Input: part model. Units: mm. Frame: model coordinates. Face numbers are marked on the shaded views. A direction names the side the tool comes from. Coordinates: 2 decimals unless noted, no trailing zeros. Loops run counter-clockwise (first coordinate to the right, second up) from the corner with the lowest first, then second, coordinate; pieces in that order, holes last.
Item 1: Reachability of the marked faces 1 and 2 from +Z, -Z, +X, -X, +Y, -Y: full face, straight path, thin tool, end or side. Return the list, or none.
Item 2: Pull-direction query (X, two-part tool) for the marked faces 3, 4 and 5; classes: released by +X, released by -X, zero draft, split by the parting line, or undercut.
Item 3: Contact query for flat-ended pins moving along their axis: P1, Ø8, axis at y = -20, z = -16, coming from the +X side; P2, Ø4, axis at x = -25, z = -6.5, coming from the -Y side; P3, Ø10, axis at y = -19.5, z = -11.5, coming from the +X side. Output: stop coordinate, or through.
Item 4: Section D-D on x = 13.5. Return loops of the section in (y, z).
Item 5: Section B-B on y = 15. Return loops of the section in (x, z).
Item 6: Section C-C on x = 38. Return loops of the section in (y, z).
Item 7: Section A-A on y = 0. Return loops of the section in (x, z), and give its area (3 significant figures).
Item 8: Ray query, line 1 along Y through (x, z) = (0, -14.5); line 2 along Z through (x, y) = (30, 18); line 3 along Y through (x, z) = (-7, -11). Return the intervals inside material, ascending.
```python
from build123d import *

# Parameters (mm, degrees)
SKETCH1_R                = 40
BOSS_EXTRUDE1_DEPTH      = 20
SKETCH3_R                = 7
BOSS_EXTRUDE2_DEPTH      = 50
BOSS_EXTRUDE2_DEPTH_BACK = 50
SKETCH5_R                = 5
CUT_EXTRUDE2_DEPTH       = 101.0000001
SKETCH2_R                = 30
CUT_EXTRUDE3_DEPTH       = 15


with BuildPart() as part:
    # Sketch1 → Boss-Extrude1 (new body)
    with BuildSketch(Plane.XY):
        Circle(SKETCH1_R)
    extrude(amount=-BOSS_EXTRUDE1_DEPTH)

    # Sketch3 → Boss-Extrude2 (add, two sides)
    with BuildSketch(Plane(origin=(0, 0, 0), x_dir=(0, 0, -1), z_dir=(1, 0, 0))) as boss_extrude2_sk:
        with Locations((10, 18)):
            Circle(SKETCH3_R)
    extrude(amount=BOSS_EXTRUDE2_DEPTH)
    extrude(boss_extrude2_sk.sketch, amount=-BOSS_EXTRUDE2_DEPTH_BACK)

    # Sketch5 → Cut-Extrude2 (cut, through all)
    with BuildSketch(Plane(origin=(50, 0, 0), x_dir=(0, 0, -1), z_dir=(1, 0, 0))):
        with Locations((10, 18)):
            Circle(SKETCH5_R)
    extrude(amount=-CUT_EXTRUDE2_DEPTH, mode=Mode.SUBTRACT)

    # Sketch2 → Cut-Extrude3 (cut)
    with BuildSketch(Plane.XY):
        Circle(SKETCH2_R)
    extrude(amount=-CUT_EXTRUDE3_DEPTH, mode=Mode.SUBTRACT)


solid = part.part
```
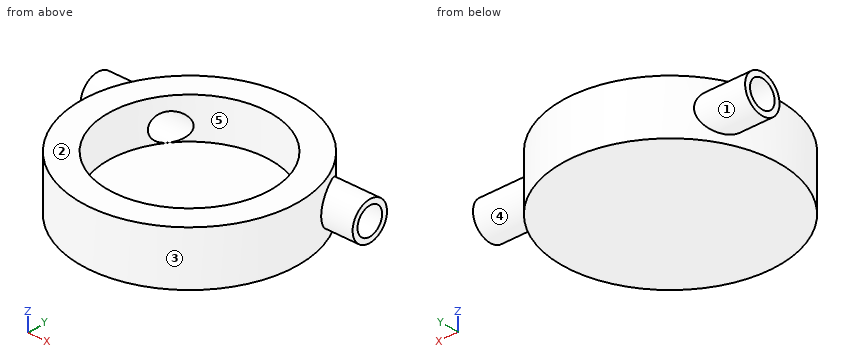
Results found:
1. face 1: -X
1. face 2: +Z, +X, -X, +Y, -Y
2. face 3: split by the parting line
2. face 4: zero draft
2. face 5: undercut
3. P1: stops at x = 36.66
3. P2: stops at y = -32.73
3. P3: stops at x = 37.28
4. outline: (-37.65, -20) - (37.65, -20) - (37.65, 0) - (26.79, 0) - (26.79, -15) - (-26.79, -15) - (-26.79, 0) - (-37.65, 0) - close
5. outline: (-50, -16.32) - (-37.08, -16.32) - (-37.08, -20) - (37.08, -20) - (37.08, -16.32) - (50, -16.32) - (50, -14) - (25.98, -14) - (25.98, -15) - (-25.98, -15) - (-25.98, -14) - (-50, -14) - close; (-50, -6) - (-25.98, -6) - (-25.98, 0) - (-37.08, 0) - (-37.08, -3.68) - (-50, -3.68) - close; (25.98, -6) - (50, -6) - (50, -3.68) - (37.08, -3.68) - (37.08, 0) - (25.98, 0) - close
6. outline: (-12.49, -20) - (12.49, -20) - (12.49, -14.32) arc R7 ccw (long way) to (12.49, -5.68) - (12.49, 0) - (-12.49, 0) - close; hole circle Ø10 at (18, -10)
7. outline: (-40, -20) - (40, -20) - (40, 0) - (30, 0) - (30, -15) - (-30, -15) - (-30, 0) - (-40, 0) - close
7. area: 700 mm2
8. line 1: y = -40 to -30, 30 to 40
8. line 2: z = -20 to -15, -5 to 0
8. line 3: y = -39.38 to -29.17, 29.17 to 39.38
